Could you check a few things on this drawing? It's one solid part, dimensions in mm from its lowest x, y, z. A direction names the side the tool comes from. Give positions to 0.01 mm unless a question says otherwise; leave off trailing zeros. Loops run counter-clockwise (first coordinate to the right, second up) from the corner with the lowest first, then second, coordinate; pieces in that order, holes last. Notation, with made-up numbers: (36, 31.25) - (62, 31.25) arc R7 ccw to (62, 41.25) - close; hole circle Ø5 at (4, -24). An arc over 180 degrees is marked (long way). Write item = value, one per line.
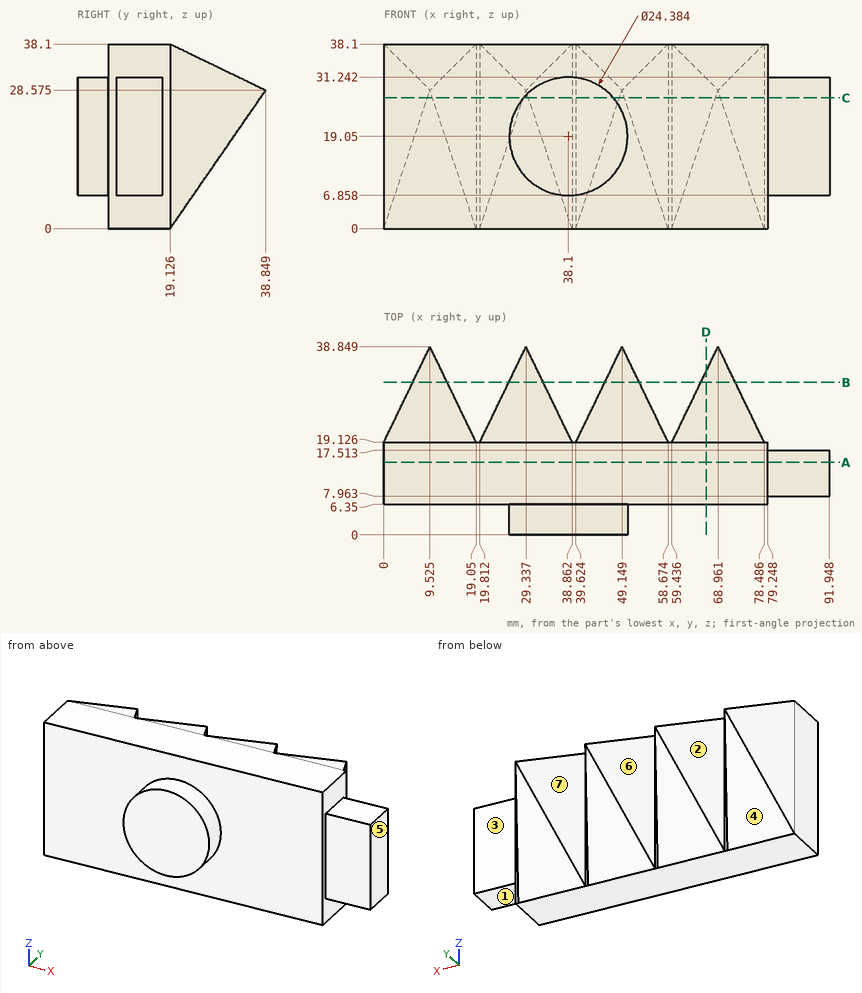
Q1. I need wall thicknesses on L1, parallel to X at y = 31.5, z = 21.5 (1 decimal); L2, parallel to X at y = 26.5, z = 13 (1 decimal); L3, parallel to Y at x = 82, z = 9. Which ranges of each line are inside material? Lowest first, please.
Output:
L1 = 6 to 13.1, 25.8 to 32.9, 45.6 to 52.7, 65.4 to 72.5
L2 = 3.6 to 15.5, 23.4 to 35.3, 43.2 to 55.1, 63 to 74.9
L3 = 7.96 to 17.51
Q2. Imagine slicing it at C-C, the plane z = 27. Write out the boundary of the cut face in (x, y).
Output:
outline = (0, 6.35) - (28.86, 6.35) - (28.86, 0) - (47.34, 0) - (47.34, 6.35) - (79.25, 6.35) - (79.25, 7.96) - (91.95, 7.96) - (91.95, 17.51) - (79.25, 17.51) - (79.25, 19.13) - (78.49, 19.13) - (69.49, 37.76) - (68.44, 37.76) - (59.44, 19.13) - (58.67, 19.13) - (49.67, 37.76) - (48.62, 37.76) - (39.62, 19.13) - (38.86, 19.13) - (29.86, 37.76) - (28.81, 37.76) - (19.81, 19.13) - (19.05, 19.13) - (10.05, 37.76) - (9, 37.76) - (0, 19.13) - close
Q3. Imagine slicing it at A-A, the plane y = 15. Write out the boundary of the cut face in (x, z), then the cut area to 3 significant figures.
Output:
outline = (0, 0) - (79.25, 0) - (79.25, 6.86) - (91.95, 6.86) - (91.95, 31.24) - (79.25, 31.24) - (79.25, 38.1) - (0, 38.1) - close
area = 3,330 mm2
Q4. Imagine slicing it at B-B, the plane y = 31.5. Write out the boundary of the cut face in (x, z).
Output:
outline = (5.98, 17.93) - (13.07, 17.93) - (13.07, 32.12) - (5.98, 32.12) - close; (25.79, 17.93) - (32.89, 17.93) - (32.89, 32.12) - (25.79, 32.12) - close; (45.6, 17.93) - (52.7, 17.93) - (52.7, 32.12) - (45.6, 32.12) - close; (65.41, 17.93) - (72.51, 17.93) - (72.51, 32.12) - (65.41, 32.12) - close
Q5. Imagine slicing it at D-D, the plane x = 66.5. Write out the boundary of the cut face in (y, z).
Output:
outline = (6.35, 0) - (19.13, 0) - (33.75, 21.19) - (33.75, 31.04) - (19.13, 38.1) - (6.35, 38.1) - close
Q6. Which directions (+Z, -Z, +X, -X, +Y, -Y) give clear straight access to the entire face, cutting with the end or side of a thin tool? Please do the marked faces 1, 2 and 3.
Output:
face_1 = -Z, +X, +Y, -Y
face_2 = +Z, -Z, +Y
face_3 = +Z, -Z, +X, +Y
Q7. For pin 1 (5 mm diameter, centred on x = 88, y = 12, fed in from -Z); pin 2 (0.8 mm diameter, centred on x = 59, z = 24, fed in from +Y); pin 3 (10 mm diameter, centred on x = 84, z = 13, fed in from -Y); pin 4 (10.5 mm diameter, centred on x = 83.5, y = 10.5, fed in from +Z), each with a flat end and sliding along its axis, tell me the tip position at first contact or that it passes through.
Output:
pin_1 = 6.86
pin_2 = 19.28
pin_3 = 6.35
pin_4 = 38.1
Q8. We'd pull the mould along X, two halves only. Please class the marked faces 4, 5, 6 and 7: released by +X, released by -X, zero draft, split by the parting line, or undercut.
Output:
face_4 = zero draft
face_5 = released by +X
face_6 = undercut
face_7 = undercut
